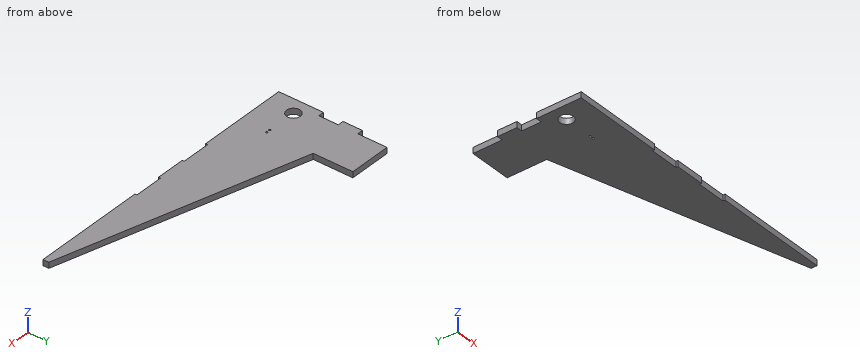
from build123d import *

# Parameters (mm, degrees)
EXTRUDE_1_DEPTH      = 0.5
EXTRUDE_2_DEPTH      = 109.5
SKETCH_8_W           = 60
SKETCH_8_H           = 8
SKETCH_8_W_2         = 60.000005443
CUT_EXTRUDE_2_DEPTH  = 10
CUT_EXTRUDE_3_DEPTH  = 10
EXTRUDE_4_DEPTH      = 2.5
FILLET_3_R           = 0.25
FILLET_4_R           = 0.25
SKETCH_7_R           = 3.5
SKETCH_7_R_2         = 0.5
CUT_EXTRUDE_4_DEPTH  = 244
SKETCH_11_W          = 306.812384231
SKETCH_11_H          = 135.84704279
CUT_EXTRUDE_6_DEPTH  = 266
SKETCH_15_W          = 3
SKETCH_15_H          = 15
SKETCH_15_H_2        = 10
CUT_EXTRUDE_9_DEPTH  = 3
SKETCH_16_W          = 15
SKETCH_16_H          = 3
CUT_EXTRUDE_10_DEPTH = 1


with BuildPart() as part:
    # Sketch 1 → Extrude 1 (new body)
    with BuildSketch(Plane.XY):
        Polygon((0, -1.078212291), (0, -59.078212291), (150, -59.078212291), (150, -56.078212291), (24.720670391, -21.433997855), (24.720670391, -1.078212291), align=None)
    extrude(amount=EXTRUDE_1_DEPTH)

    # Sketch 2 → Extrude 2 (add)
    with BuildSketch(Plane(origin=(0, 0, 0), x_dir=(-1, 0, 0), z_dir=(0, 0, -1))):
        with BuildLine():
            Line((0, -1.078212291), (-2.47, -1.078212291))
            Line((-2.47, -1.078212291), (-2.47, -54.078212291))
            Line((-2.47, -54.078212291), (-149.757622023, -58.570819212))
            ThreePointArc((-149.757622023, -58.570819212), (-149.929451255, -58.64664195), (-150, -58.820702994))
            Line((-150, -58.820702994), (-150, -58.828212291))
            ThreePointArc((-150, -58.828212291), (-149.926776695, -59.004988986), (-149.75, -59.078212291))
            Line((-149.75, -59.078212291), (0, -59.078212291))
            Line((0, -59.078212291), (0, -1.078212291))
        make_face()
    extrude(amount=EXTRUDE_2_DEPTH)

    # Mirror 3: part across plane


with BuildPart() as part_1:
    add(part.part)
    add(part.part.mirror(Plane(origin=(149.75, -58.820702994, -109.5), x_dir=(1, 0, 0), z_dir=(0, 0, 1))))

    # Sketch 8 → Cut-Extrude 2 (cut)
    with BuildSketch(Plane(origin=(-1.645679091, -53.952674733, 0), x_dir=(0.9995351300973986, -0.030488091136977483, 0), z_dir=(0.030488091136977483, 0.9995351300973986, 0))):
        with Locations((121.473716686, 5)):
            Rectangle(SKETCH_8_W, SKETCH_8_H)
        with Locations((121.473713965, 15)):
            Rectangle(SKETCH_8_W_2, SKETCH_8_H)
        with Locations((121.473713965, 24.947368421)):
            Rectangle(SKETCH_8_W_2, SKETCH_8_H)
        with Locations((121.473713965, 34.894736842)):
            Rectangle(SKETCH_8_W_2, SKETCH_8_H)
        with Locations((121.473713965, 44.842105263)):
            Rectangle(SKETCH_8_W_2, SKETCH_8_H)
        with Locations((121.473713965, 54.789473684)):
            Rectangle(SKETCH_8_W_2, SKETCH_8_H)
        with Locations((121.473713965, 64.736842105)):
            Rectangle(SKETCH_8_W_2, SKETCH_8_H)
        with Locations((121.473713965, 74.684210526)):
            Rectangle(SKETCH_8_W_2, SKETCH_8_H)
        with Locations((121.473713965, 84.631578947)):
            Rectangle(SKETCH_8_W_2, SKETCH_8_H)
        with Locations((121.473713965, 94.578947368)):
            Rectangle(SKETCH_8_W_2, SKETCH_8_H)
        with Locations((121.473713965, 104.526315789)):
            Rectangle(SKETCH_8_W_2, SKETCH_8_H)
        with Locations((121.473713965, 114.473684211)):
            Rectangle(SKETCH_8_W_2, SKETCH_8_H)
        with Locations((121.473713965, 124.421052632)):
            Rectangle(SKETCH_8_W_2, SKETCH_8_H)
        with Locations((121.473713965, 134.368421053)):
            Rectangle(SKETCH_8_W_2, SKETCH_8_H)
        with Locations((121.473713965, 144.315789474)):
            Rectangle(SKETCH_8_W_2, SKETCH_8_H)
        with Locations((121.473713965, 154.263157895)):
            Rectangle(SKETCH_8_W_2, SKETCH_8_H)
        with Locations((121.473713965, 164.210526316)):
            Rectangle(SKETCH_8_W_2, SKETCH_8_H)
        with Locations((121.473713965, 174.157894737)):
            Rectangle(SKETCH_8_W_2, SKETCH_8_H)
        with Locations((121.473713965, 184.105263158)):
            Rectangle(SKETCH_8_W_2, SKETCH_8_H)
        with Locations((121.473713965, 194.052631579)):
            Rectangle(SKETCH_8_W_2, SKETCH_8_H)
        with Locations((121.473713965, 204)):
            Rectangle(SKETCH_8_W_2, SKETCH_8_H)
        with Locations((121.473716686, 214)):
            Rectangle(SKETCH_8_W, SKETCH_8_H)
    extrude(amount=-CUT_EXTRUDE_2_DEPTH, mode=Mode.SUBTRACT)

    # Sketch 9 → Cut-Extrude 3 (cut)
    with BuildSketch(Plane(origin=(-1.645679091, -53.952674733, 0), x_dir=(0.9995351300973986, -0.030488091136977483, 0), z_dir=(0.030488091136977483, 0.9995351300973986, 0))):
        Polygon((151.639987162, 219), (153.085665737, 219), (154.855962757, 1), (151.716207414, 1), (151.473716686, 1), (151.473716686, 219), align=None)
    extrude(amount=-CUT_EXTRUDE_3_DEPTH, mode=Mode.SUBTRACT)

    # Sketch 1_3 → Extrude 4 (add)
    with BuildSketch(Plane.XY):
        Polygon((0, -1.078212291), (0, -59.078212291), (150, -59.078212291), (150, -56.078212291), (24.720670391, -21.433997855), (24.720670391, -1.078212291), align=None)
    extrude_4 = extrude(amount=-EXTRUDE_4_DEPTH)

    # Fillet 3
    fillet_3_edges = [part_1.edges().sort_by_distance(p)[0] for p in [
        (149.757622023, -58.570819212, -218.5),
        (149.757622023, -58.570819212, -209),
        (149.757622023, -58.570819212, -199.026315789),
        (149.757622023, -58.570819212, -189.078947368),
        (149.757622023, -58.570819212, -179.131578947),
        (149.757622023, -58.570819212, -169.184210526),
        (149.757622023, -58.570819212, -159.236842105),
        (149.757622023, -58.570819212, -149.289473684),
        (149.757622023, -58.570819212, -139.342105263),
        (149.757622023, -58.570819212, -129.394736842),
        (149.757622023, -58.570819212, -119.447368421),
        (149.757622023, -58.570819212, -109.5),
        (149.757622023, -58.570819212, -99.552631579),
        (149.757622023, -58.570819212, -89.605263158),
        (149.757622023, -58.570819212, -79.657894737),
        (149.757622023, -58.570819212, -69.710526316),
        (149.757622023, -58.570819212, -59.763157895),
        (149.757622023, -58.570819212, -49.815789474),
        (149.757622023, -58.570819212, -39.868421053),
        (149.757622023, -58.570819212, -29.921052632),
        (149.757622023, -58.570819212, -19.973684211),
        (149.757622023, -58.570819212, -10),
    ]]
    fillet(fillet_3_edges, radius=FILLET_3_R)

    # Fillet 4
    fillet_4_edges = [part_1.edges().sort_by_distance(p)[0] for p in [
        (149.742145382, -59.078212291, -218.5),
        (149.742145382, -59.078212291, -209),
        (149.742145382, -59.078212291, -199.026315789),
        (149.742145382, -59.078212291, -189.078947368),
        (149.742145382, -59.078212291, -179.131578947),
        (149.742145382, -59.078212291, -169.184210526),
        (149.742145382, -59.078212291, -159.236842105),
        (149.742145382, -59.078212291, -149.289473684),
        (149.742145382, -59.078212291, -139.342105263),
        (149.742145382, -59.078212291, -129.394736842),
        (149.742145382, -59.078212291, -119.447368421),
        (149.742145382, -59.078212291, -109.5),
        (149.742145382, -59.078212291, -99.552631579),
        (149.742145382, -59.078212291, -89.605263158),
        (149.742145382, -59.078212291, -79.657894737),
        (149.742145382, -59.078212291, -69.710526316),
        (149.742145382, -59.078212291, -59.763157895),
        (149.742145382, -59.078212291, -49.815789474),
        (149.742145382, -59.078212291, -39.868421053),
        (149.742145382, -59.078212291, -29.921052632),
        (149.742145382, -59.078212291, -19.973684211),
        (149.742145382, -59.078212291, -10),
    ]]
    fillet(fillet_4_edges, radius=FILLET_4_R)

    # Mirror 4: Extrude 4 across plane
    add(extrude_4.mirror(Plane.XY.offset(-109.5)))

    # Sketch 7 → Cut-Extrude 4 (cut)
    with BuildSketch(Plane.XY.offset(0.5)):
        with Locations(Location((8, -45.078212291, 0), (0, 0, 180))):
            Circle(SKETCH_7_R)
        with Locations(Location((25, -45.078212291, 0), (0, 0, 180))):
            Circle(SKETCH_7_R_2)
        with Locations(Location((23, -45.078212291, 0), (0, 0, 180))):
            Circle(SKETCH_7_R_2)
    extrude(amount=-CUT_EXTRUDE_4_DEPTH, mode=Mode.SUBTRACT)

    # Sketch 11 → Cut-Extrude 6 (cut)
    with BuildSketch(Plane(origin=(150, 0, 0), x_dir=(0, 0, -1), z_dir=(1, 0, 0))):
        with Locations((155.906192116, 8.845309104)):
            Rectangle(SKETCH_11_W, SKETCH_11_H)
    extrude(amount=-CUT_EXTRUDE_6_DEPTH, mode=Mode.SUBTRACT)

    # Sketch 15 → Cut-Extrude 9 (cut)
    with BuildSketch(Plane.ZY):
        with Locations((-1, -8.578212291)):
            Rectangle(SKETCH_15_W, SKETCH_15_H)
        with Locations((-1, -31.078212291)):
            Rectangle(SKETCH_15_W, SKETCH_15_H_2)
    extrude(amount=-CUT_EXTRUDE_9_DEPTH, mode=Mode.SUBTRACT)

    # Sketch 16 → Cut-Extrude 10 (cut)
    with BuildSketch(Plane(origin=(0, -59.078212291, 0), x_dir=(-1, 0, 0), z_dir=(0, -1, 0))):
        with Locations((-83.973716686, 1)):
            Rectangle(SKETCH_16_W, SKETCH_16_H)
        with Locations((-53.973716686, 1)):
            Rectangle(SKETCH_16_W, SKETCH_16_H)
    extrude(amount=-CUT_EXTRUDE_10_DEPTH, mode=Mode.SUBTRACT)


solid = part_1.part
Work out the finished part from the listing and answer in its coordinate system (mm). Give positions to 0.01 mm unless a question says otherwise; leave off trailing zeros. Order: outer loops, then holes, each group sorted by start corner. A loop starts at its lowest first (then second) coordinate and runs counter-clockwise, first axis right, second up. Notation, with made-up numbers: M 33,81 L 56,81 A10 ccw 56,94 Z; hole C -40,7.5 d1. An arc over 180 degrees is marked long. Return JSON: item names as keys, results as strings.
Q1. Find section C-C, the plane y = -5. Write down the section's boundary in (x, z).
Answer below:
{"outline": "M 3,-2.5 L 24.72,-2.5 L 24.72,0.5 L 3,0.5 Z"}
Q2. Find section A-A, the plane x = 8. Write down the section's boundary in (y, z), and give its area (3 significant figures).
Answer below:
{"outline": "M -59.08,-2.5 L -48.58,-2.5 L -48.58,0.5 L -59.08,0.5 Z; M -41.58,-2.5 L -1.08,-2.5 L -1.08,0.5 L -41.58,0.5 Z", "area": "153 mm^2"}
Q3. Find section B-B, the plane z = -1.4. Write down the section's boundary in (x, y), and give its area (3 significant figures).
Answer below:
{"outline": "M 0,-59.08 L 46.47,-59.08 L 46.47,-58.08 L 61.47,-58.08 L 61.47,-59.08 L 76.47,-59.08 L 76.47,-58.08 L 91.47,-58.08 L 91.47,-59.08 L 150,-59.08 L 150,-56.08 L 24.72,-21.43 L 24.72,-1.08 L 3,-1.08 L 3,-16.08 L 0,-16.08 L 0,-26.08 L 3,-26.08 L 3,-36.08 L 0,-36.08 Z; hole C 8,-45.08 d7; hole C 23,-45.08 d1; hole C 25,-45.08 d1", "area": "3,830 mm^2"}
Q4. Find the intervals of material crossed by line 1 along Y through (x, z) = (23, -0.3); line 2 along Y through (x, z) = (8, -0.35); line 3 along X through (y, z) = (-7, -1.85), in increasing order. Write a range as [from, to].
Answer below:
{"line 1": "y = [-59.08, -45.58], [-44.58, -1.08]", "line 2": "y = [-59.08, -48.58], [-41.58, -1.08]", "line 3": "x = [3, 24.72]"}
Q5. Each of these flat-tipped pins is pushed along its axis until it touches: pin 1 (0.5 mm diameter, centred on y = -58.5, z = -1.5, fed in from -X); pin 2 (1.5 mm diameter, centred on y = -6.5, z = -1.5, fed in from -X); pin 3 (1.5 mm diameter, centred on y = -10.5, z = -0.5, fed in from +X). Where does it stop, or does it pass through?
Answer below:
{"pin 1": "stops at x = 0", "pin 2": "stops at x = 3", "pin 3": "stops at x = 24.72"}
Q6. Find section D-D, the plane x = 93. Write down the section's boundary in (y, z), and give its area (3 significant figures).
Answer below:
{"outline": "M -59.08,-2.5 L -40.32,-2.5 L -40.32,0.5 L -59.08,0.5 Z", "area": "56.3 mm^2"}
